Check sheet for the modelled part. Datum: model origin and axes. Units: mm. Give positions to 0.01 mm unless a question says otherwise; leave off trailing zeros. Write each loop counter-clockwise with the first axis right and the second up, starting at its lowest first coordinate (ties: lowest second). Pieces come first, ordered by that corner, then holes. Notation, with made-up numbers: (-4.5, -35) -> (19.5, -35) arc R18 ccw to (19.5, -11) -> close; hole circle Ø5 at (73.25, -16.5). An arc over 180 degrees is marked (long way). Answer as a JSON object with one key per item and string values.
from build123d import *

# Parameters (mm, degrees)
SKETCH2_R           = 13.2
BOSS_EXTRUDE1_DEPTH = 2
SKETCH3_R           = 1.9
CUT_EXTRUDE1_DEPTH  = 2
SKETCH4_R           = 5
CUT_EXTRUDE2_DEPTH  = 2
CIRPATTERN1_COUNT   = 4
FILLET2_R           = 1


with BuildPart() as part:
    # Sketch2 → Boss-Extrude1 (new body)
    with BuildSketch(Plane(origin=(0, 0, 0), x_dir=(1, 0, 0), z_dir=(0, 1, 0))):
        with Locations(Location((0, 0, 0), (0, 0, 270))):
            Circle(SKETCH2_R)
    extrude(amount=BOSS_EXTRUDE1_DEPTH)

    # Sketch3 → Cut-Extrude1 (cut)
    with BuildSketch(Plane(origin=(0, 2, 0), x_dir=(1, 0, 0), z_dir=(0, 1, 0))):
        with Locations(Location((0, 10, 0), (0, 0, 270))):
            Circle(SKETCH3_R)
    cut_extrude1 = extrude(amount=-CUT_EXTRUDE1_DEPTH, mode=Mode.SUBTRACT)

    # Sketch4 → Cut-Extrude2 (cut)
    with BuildSketch(Plane(origin=(0, 2, 0), x_dir=(1, 0, 0), z_dir=(0, 1, 0))):
        with Locations(Location((0, 0, 0), (0, 0, 270))):
            Circle(SKETCH4_R)
    extrude(amount=-CUT_EXTRUDE2_DEPTH, mode=Mode.SUBTRACT)

    # CirPattern1: Cut-Extrude1 ×4 about axis
    cirpattern1_axis = Axis((0, 0, 0), (0, 1, 0))
    for i in range(1, CIRPATTERN1_COUNT):
        add(cut_extrude1.rotate(cirpattern1_axis, i * 360 / CIRPATTERN1_COUNT), mode=Mode.SUBTRACT)

    # Fillet2
    fillet2_edges = [part.edges().sort_by_distance(p)[0] for p in [
        (0, 0, -5),
        (0, 2, -5),
    ]]
    fillet(fillet2_edges, radius=FILLET2_R - 0.0001)  # a hair under: the kernel refuses the full size


solid = part.part
1. Sectioned sample at C-C, the plane x = -10. Enter the section's corners in (y, z).
Determined:
{"outline": "(0, -8.62) -> (2, -8.62) -> (2, -1.9) -> (0, -1.9) -> close; (0, 1.9) -> (2, 1.9) -> (2, 8.62) -> (0, 8.62) -> close"}
2. Mould release check, pull along Z, two halves, no side actions. Record for faces 1 (the face through (-8, 1, -10.5)), 2 (the face through (-8.188, 1.014, -0.571)), 3 (the face through (-3, 2, 6)): released by +Z, released by -Z, zero draft, split by the parting line, or undercut.
Determined:
{"face 1": "split by the parting line", "face 2": "undercut", "face 3": "zero draft"}
3. Sectioned sample at A-A, the plane z = 0. State how many separate pieces and enclosed holes the cut face has, plus the area to 3 significant figures.
Determined:
{"separate pieces": "4", "enclosed holes": "0", "area": "16.7 mm^2"}
4. Go/stop test with flat-tipped pins: P1, Ø5, axis at x = 0, z = 10, coming from the +Y side; P2, Ø3, axis at x = -10, z = 0, coming from the +Y side. Record where each tip stops, or that it passes through.
Determined:
{"P1": "y = 2", "P2": "through"}
5. Scan lines: L1, parallel to Z at x = 1.5, y = 1.8; L2, parallel to Z at x = -10.5, y = 0.6; L3, parallel to Z at x = 4.5, y = 0.55. Record each from-to range of solid material in increasing order. Write a range as [from, to].
Determined:
{"L1": "[-13.11, -11.17], [-8.83, -5.19], [5.19, 8.83], [11.17, 13.11]", "L2": "[-8, -1.83], [1.83, 8]", "L3": "[-12.41, -2.41], [2.41, 12.41]"}
6. Sectioned sample at D-D, the plane z = -11. Enter the section's corners in (x, y).
Determined:
{"outline": "(-7.3, 0) -> (-1.62, 0) -> (-1.62, 2) -> (-7.3, 2) -> close; (1.62, 0) -> (7.3, 0) -> (7.3, 2) -> (1.62, 2) -> close"}
